from build123d import *

# Parameters (mm, degrees)
F1_W     = 769.9375
F1_H     = 755.65
F1_W_2   = 731.8248
F1_H_2   = 717.55
F2_DEPTH = 182.5625


with BuildPart() as f2:
    # F1 (on face) → F2 (new body, symmetric)
    with BuildSketch(Plane.XZ):
        Rectangle(F1_W, F1_H)
        Rectangle(F1_W_2, F1_H_2, mode=Mode.SUBTRACT)
    extrude(amount=F2_DEPTH, both=True)


solid = f2.part
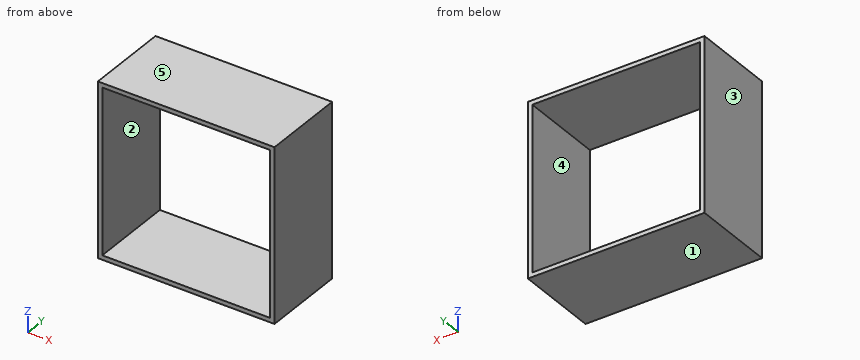
Check sheet for the modelled part. Datum: model origin and axes. Units: mm. Face numbers are marked on the shaded views. A direction names the side the tool comes from. Give positions to 0.01 mm unless a question says otherwise; leave off trailing zeros. Loops run counter-clockwise (first coordinate to the right, second up) from the corner with the lowest first, then second, coordinate; pieces in that order, holes last. Notation, with made-up numbers: M -39,44 L -22,44 A14 ccw -22,71 Z; hole C 79,37 d11. An arc over 180 degrees is marked long. Use a Markdown table: item, result. Add a question column.
Q1. Tool access check on the marked faces 4 and 5. Record the directions out of +Z, -Z, +X, -X, +Y, -Y that give a thin tool (end or side, any length) a straight path to the whole face; none if there is none.
Q2. Sectioned sample at A-A, the plane x = -17.5. Record the cut outline in (y, z) (1 decimal), then the cut area to 3 significant figures.
Q3. Sectioned sample at B-B, the plane z = -3. Record the cut outline in (x, y), then the cut area to 3 significant figures.
Q4. Mould release check, pull along X, two halves, no side actions. Record for the marked faces 1, 2 and 3: pulls with the +X half, pulls with the -X half, needs draft (parallel to the pull), parting line crosses it, or undercut.
Q5. Sectioned sample at C-C, the plane y = -76.5. Record the cut outline in (x, z) (3 decimals).
Q6. Scan lines: line 1 along Z through (x, y) = (-58, 81.5) (3 decimals); line 2 along X through (y, z) = (-32, -96.5). Record each from-to range of solid material in increasing order. Write a range as [from, to].
Verdict:
| question | item | result |
|---|---|---|
| 1 | face 4 | +Y, -Y |
| 1 | face 5 | +Z, +X, -X, +Y, -Y |
| 2 | outline | M -182.6,-377.8 L 182.6,-377.8 L 182.6,-358.8 L -182.6,-358.8 Z; M -182.6,358.8 L 182.6,358.8 L 182.6,377.8 L -182.6,377.8 Z |
| 2 | area | 13,900 mm^2 |
| 3 | outline | M -384.97,-182.56 L -365.91,-182.56 L -365.91,182.56 L -384.97,182.56 Z; M 365.91,-182.56 L 384.97,-182.56 L 384.97,182.56 L 365.91,182.56 Z |
| 3 | area | 13,900 mm^2 |
| 4 | face 1 | needs draft |
| 4 | face 2 | undercut |
| 4 | face 3 | pulls with the -X half |
| 5 | outline | M -384.969,-377.825 L 384.969,-377.825 L 384.969,377.825 L -384.969,377.825 Z; hole M -365.912,-358.775 L 365.912,-358.775 L 365.912,358.775 L -365.912,358.775 Z |
| 6 | line 1 | [-377.825, -358.775], [358.775, 377.825] |
| 6 | line 2 | [-384.97, -365.91], [365.91, 384.97] |
